Model file for the job. Use its own axes, mm. Face numbers are marked on the shaded views. Coordinates: 2 decimals unless noted, no trailing zeros. Write each loop counter-clockwise with the first axis right and the second up, starting at its lowest first coordinate (ties: lowest second). Pieces come first, ordered by that corner, then holes. Notation, with made-up numbers: (-22.75, 36.25) -> (4.25, 36.25) arc R29 ccw to (4.25, 66.25) -> close; hole circle Ø9 at (11.25, 88.25). An arc over 180 degrees is marked (long way). Answer as a JSON object with one key per item and string values. Group by question number.
from build123d import *

# Parameters (mm, degrees)
SKETCH_1_R      = 1.5
EXTRUDE_1_DEPTH = 2
FILLET_1_R      = 1


with BuildPart() as part:
    # 草图1 → 凸台-拉伸1 (new body)
    with BuildSketch(Plane.XY):
        Polygon((0, 10), (14, 10), (14, -6.402050808), (6.272169318, -10.863715932), (0, 0), align=None)
        with Locations((7, 5)):
            Circle(SKETCH_1_R, mode=Mode.SUBTRACT)
        with Locations((7, -4.67)):
            Circle(SKETCH_1_R, mode=Mode.SUBTRACT)
    extrude(amount=EXTRUDE_1_DEPTH)

    # 圆角1
    fillet_1_edges = [part.edges().sort_by_distance(p)[0] for p in [
        (0, 10, 1),
        (14, 10, 1),
        (14, -6.402050808, 1),
        (6.272169318, -10.863715932, 1),
        (0, 0, 1),
    ]]
    fillet(fillet_1_edges, radius=FILLET_1_R)


solid = part.part
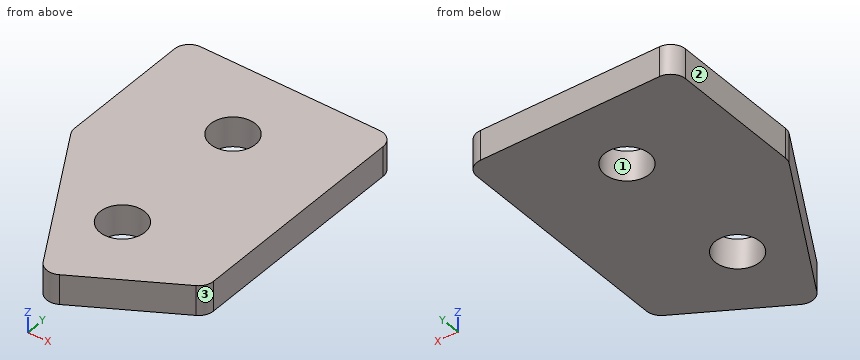
(1) Cut at D-D on x = 1.75. List the corners of the cut face in (y, z).
(2) Cut at B-B on z = 0.65. List the corners of the cut face in (x, y).
(3) Wall check: probe 1 along Y at (x, z) = (7, 1.2); probe 2 along X at (y, z) = (6.25, 0.1); probe 3 along X at (y, z) = (4.5, 0.25). Give the ranges that are in metal, low to high.
(4) Pin check, flat tip, straight feed: pin 1 (2.5 mm diameter, centred on x = 7, y = -4.67, fed in from -Z). Stop position of the tip, or through.
(5) Cut at C-C on y = -4.67. List the corners of the cut face in (x, z), plus the area to 3 significant figures.
(6) Pull direction Y, two halves, no side cores. Call the marked faces 1, 2 and 3: released by +Y, released by -Y, zero draft, split by the parting line, or undercut.
(7) Cut at A-A on y = 5. List the corners of the cut face in (x, z), plus the area to 3 significant figures.
Results found:
{
 "1": {"outline": "(-3.03, 0) -> (10, 0) -> (10, 2) -> (-3.03, 2) -> close"},
 "2": {"outline": "(0, 0.27) arc R1 ccw to (0.13, -0.23) -> (5.77, -10) arc R1 ccw to (7.14, -10.36) -> (13.5, -6.69) arc R1 ccw to (14, -5.82) -> (14, 9) arc R1 ccw to (13, 10) -> (1, 10) arc R1 ccw to (0, 9) -> close; hole circle Ø3 at (7, -4.67); hole circle Ø3 at (7, 5)"},
 "3": {"probe 1": "y = -10.43 to -6.17, -3.17 to 3.5, 6.5 to 10", "probe 2": "x = 0 to 6.17, 7.83 to 14", "probe 3": "x = 0 to 5.59, 8.41 to 14"},
 "4": {"pin 1": "passes through"},
 "5": {"outline": "(2.7, 0) -> (5.5, 0) -> (5.5, 2) -> (2.7, 2) -> close; (8.5, 0) -> (14, 0) -> (14, 2) -> (8.5, 2) -> close", "area": "16.6 mm²"},
 "6": {"face 1": "undercut", "face 2": "zero draft", "face 3": "released by -Y"},
 "7": {"outline": "(0, 0) -> (5.5, 0) -> (5.5, 2) -> (0, 2) -> close; (8.5, 0) -> (14, 0) -> (14, 2) -> (8.5, 2) -> close", "area": "22.0 mm²"}
}
